from build123d import *

# Parameters (mm, degrees)
F0_W     = 50
F0_H     = 12
F1_DEPTH = 9
F2_R     = 1.5
F3_DEPTH = 12
F4_W     = 27
F4_H     = 5
F5_DEPTH = 12.5
F7_DEPTH = 9


with BuildPart() as f1:
    # F0 (on Top) → F1 (new body)
    with BuildSketch(Plane.XY):
        with Locations((25, 6)):
            Rectangle(F0_W, F0_H)
    extrude(amount=F1_DEPTH)

    # F2 (on face) → F3 (cut)
    with BuildSketch(Plane.XZ):
        with Locations((5, 4.5)):
            Circle(F2_R)
        with Locations((45, 4.5)):
            Circle(F2_R)
    extrude(amount=-F3_DEPTH, mode=Mode.SUBTRACT)

    # F4 (on face) → F5 (cut)
    with BuildSketch(Plane(origin=(0, 12, 0), x_dir=(-1, 0, 0), z_dir=(0, 1, 0))):
        with Locations((-25, 4.5)):
            Rectangle(F4_W, F4_H)
    extrude(amount=-F5_DEPTH, mode=Mode.SUBTRACT)

    # F6 (on face) → F7 (cut)
    with BuildSketch(Plane.XY.offset(9)):
        with BuildLine():
            ThreePointArc((15.25, 12), (25, 2.25), (34.75, 12))
            Line((34.75, 12), (15.25, 12))
        make_face()
    extrude(amount=-F7_DEPTH, mode=Mode.SUBTRACT)


solid = f1.part
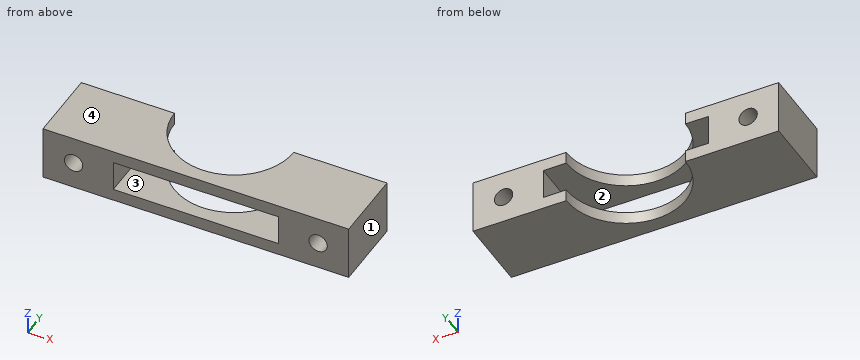
Read the model definition and answer for the solid it produces. Units are mm, in the model's axes. Face numbers are marked on the shaded views. Coordinates: 2 decimals unless noted, no trailing zeros. Loops run counter-clockwise (first coordinate to the right, second up) from the corner with the lowest first, then second, coordinate; pieces in that order, holes last.
Q1. The mould has two halves that part along X. Classify the marked faces 1, 2, 3 and 4: +X half, -X half, draft (parallel to the pull), parting line (faces both ways), or undercut.
Q2. Consider probe 1 along Z at (x, y) = (45, 7); probe 2 along Z at (x, y) = (25, 1.75); probe 3 along X at (y, z) = (1.5, 5.5). Determine where each line is inside the solid, lowest interval first.
Q3. This flat-tipped pin is pushed along its axis until it touches: pin 1 Ø2.5 at (x, z) = (5, 4.5) entering from -Y. Where does it stop, or does it pass through?
Q4. The part is cut by section B-B on y = 8. Write down the section's boundary in (x, z), and give its area (3 significant figures).
Q5. The part is cut by section D-D on x = 5. Write down the section's boundary in (y, z).
Q6. The part is cut by section A-A on z = 4.5. Write down the section's boundary in (x, y), and give its area (3 significant figures).
Q7. The part is cut by section C-C on x = 25. Write down the section's boundary in (y, z), and give its area (3 significant figures).
Results below:
1. face 1: +X half
1. face 2: undercut
1. face 3: undercut
1. face 4: draft
2. probe 1: z = 0 to 3, 6 to 9
2. probe 2: z = 0 to 2, 7 to 9
2. probe 3: x = 0 to 3.88, 6.12 to 11.5, 38.5 to 43.88, 46.12 to 50
3. pin 1: passes through
4. outline: (0, 0) - (16.11, 0) - (16.11, 2) - (11.5, 2) - (11.5, 7) - (16.11, 7) - (16.11, 9) - (0, 9) - close; (33.89, 0) - (50, 0) - (50, 9) - (33.89, 9) - (33.89, 7) - (38.5, 7) - (38.5, 2) - (33.89, 2) - close; hole circle Ø3 at (5, 4.5); hole circle Ø3 at (45, 4.5)
4. area: 230 mm2
5. outline: (0, 0) - (12, 0) - (12, 3) - (0, 3) - close; (0, 6) - (12, 6) - (12, 9) - (0, 9) - close
6. outline: (0, 0) - (3.5, 0) - (3.5, 12) - (0, 12) - close; (6.5, 0) - (11.5, 0) - (11.5, 12) - (6.5, 12) - close; (38.5, 0) - (43.5, 0) - (43.5, 12) - (38.5, 12) - close; (46.5, 0) - (50, 0) - (50, 12) - (46.5, 12) - close
6. area: 204 mm2
7. outline: (0, 0) - (2.25, 0) - (2.25, 2) - (0, 2) - close; (0, 7) - (2.25, 7) - (2.25, 9) - (0, 9) - close
7. area: 9.00 mm2
